Geometry check sheet. Reference: the model listing, model coordinates, mm. A direction names the side the tool comes from. Give positions to 0.01 mm unless a question says otherwise; leave off trailing zeros. Loops run counter-clockwise (first coordinate to the right, second up) from the corner with the lowest first, then second, coordinate; pieces in that order, holes last.
1. Cross-section at B-B, the plane z = 31.75. Record the cut outline in (x, y) (3 decimals).
2. Go/stop test with flat-tipped pins: pin 1 Ø1.3 at (x, z) = (-1.5, 22) entering from +Y; pin 2 Ø8 at (y, z) = (-13, 26) entering from -X; pin 3 Ø0.6 at (x, y) = (4.5, 9.5) entering from -Z; pin 4 Ø0.9 at (x, y) = (-5.5, 6) entering from +Z. Record where each tip stops, or that it passes through.
3. Tool access check on faces 1 (the flat face through (0, -17.78, -22)), 2 (the flat face through (5.25, 9, -4)), 3 (the flat face through (0, -4, 6.02)). Record the directions out of +Z, -Z, +X, -X, +Y, -Y that give a thin tool (end or side, any length) a straight path to the whole face; none if there is none.
4. Cross-section at C-C, the plane z = -31. Record the cut outline in (x, y) (3 decimals).
5. Cross-section at A-A, the plane y = 12.5. Record the cut outline in (x, z), plus the area to 3 significant figures.
6. Material ranges on L1, parallel to Z at x = -5, y = 6.5; L2, parallel to X at y = -18.6, z = 31.75, recorded low to high.
7. Cross-section at D-D, the plane y = -14.5. Record the cut outline in (x, z), plus the area to 3 significant figures.
from build123d import *

# Parameters (mm, degrees)
BOSS_EXTRUDE1_DEPTH   = 17.78
BOSS_EXTRUDE1_2_DEPTH = 17.78
BOSS_EXTRUDE1_3_DEPTH = 17.78
BOSS_EXTRUDE1_4_DEPTH = 17.78
SKETCH2_W             = 13.04
SKETCH2_H             = 12.04
BOSS_EXTRUDE2_DEPTH   = 17.78
SKETCH3_W             = 12.7
SKETCH3_H             = 76.2
SKETCH3_R             = 3.429
BOSS_EXTRUDE3_DEPTH   = 3.175
SKETCH4_OUTSIDE_W     = 32.334
SKETCH4_OUTSIDE_H     = 95.494
SKETCH4_OUTSIDE_W_2   = 12.7
SKETCH4_OUTSIDE_H_2   = 76.2
CUT_EXTRUDE2_DEPTH    = 55.722213268
CUT_EXTRUDE3_DEPTH    = 0.635


with BuildPart() as part:
    # Sketch1 → Boss-Extrude1 (new body)
    with BuildSketch(Plane(origin=(0, 0, 0), x_dir=(1, 0, 0), z_dir=(0, 1, 0))):
        Polygon((-5.25, 4.75), (-5.25, 2.718), (-6.52, 2.718), (-6.52, 6.02), (-3.218, 6.02), (-3.218, 4.75), align=None)
    extrude(amount=BOSS_EXTRUDE1_DEPTH)



with BuildPart() as body_2:
    # Sketch1 → Boss-Extrude1 2 (new body)
    with BuildSketch(Plane(origin=(0, 0, 0), x_dir=(1, 0, 0), z_dir=(0, 1, 0))):
        Polygon((6.52, 2.718), (6.52, 6.02), (3.218, 6.02), (3.218, 4.75), (5.25, 4.75), (5.25, 2.718), align=None)
    extrude(amount=BOSS_EXTRUDE1_2_DEPTH)


with BuildPart() as body_3:
    # Sketch1 → Boss-Extrude1 3 (new body)
    with BuildSketch(Plane(origin=(0, 0, 0), x_dir=(1, 0, 0), z_dir=(0, 1, 0))):
        Polygon((5.25, -2.718), (6.52, -2.718), (6.52, -6.02), (3.218, -6.02), (3.218, -4.75), (5.25, -4.75), align=None)
    extrude(amount=BOSS_EXTRUDE1_3_DEPTH)


with BuildPart() as body_4:
    # Sketch1 → Boss-Extrude1 4 (new body)
    with BuildSketch(Plane(origin=(0, 0, 0), x_dir=(1, 0, 0), z_dir=(0, 1, 0))):
        Polygon((-5.25, -2.718), (-6.52, -2.718), (-6.52, -6.02), (-3.218, -6.02), (-3.218, -4.75), (-5.25, -4.75), align=None)
    extrude(amount=BOSS_EXTRUDE1_4_DEPTH)


with BuildPart() as part_1:
    add(part.part)

    add(body_2.part)  # Boss-Extrude2 merges body 2

    add(body_3.part)  # Boss-Extrude2 merges body 3

    add(body_4.part)  # Boss-Extrude2 merges body 4
    # Sketch2 → Boss-Extrude2 (add)
    with BuildSketch(Plane(origin=(0, 0, 0), x_dir=(-1, 0, 0), z_dir=(0, -1, 0))):
        Rectangle(SKETCH2_W, SKETCH2_H)
    extrude(amount=BOSS_EXTRUDE2_DEPTH)

    # Sketch3 → Boss-Extrude3 (add)
    with BuildSketch(Plane(origin=(0, -17.78, 0), x_dir=(-1, 0, 0), z_dir=(0, -1, 0))):
        Rectangle(SKETCH3_W, SKETCH3_H)
        with Locations(Location((0, 31.75, 0), (0, 0, 90))):
            Circle(SKETCH3_R, mode=Mode.SUBTRACT)
        with Locations(Location((0, -31.75, 0), (0, 0, 270))):
            Circle(SKETCH3_R, mode=Mode.SUBTRACT)
    extrude(amount=BOSS_EXTRUDE3_DEPTH)

    # Sketch4 outside → Cut-Extrude2 (cut, through all)
    with BuildSketch(Plane.XZ.offset(20.955)):
        Rectangle(SKETCH4_OUTSIDE_W, SKETCH4_OUTSIDE_H)
        Rectangle(SKETCH4_OUTSIDE_W_2, SKETCH4_OUTSIDE_H_2, mode=Mode.SUBTRACT)
    extrude(amount=-CUT_EXTRUDE2_DEPTH, mode=Mode.SUBTRACT)

    # Sketch5 → Cut-Extrude3 (cut)
    with BuildSketch(Plane(origin=(0, -17.78, 0), x_dir=(1, 0, 0), z_dir=(0, 1, 0))):
        Polygon((-4.402938034, -19.56265828), (-3.33951656, -19.56265828), (-2.238782051, -22.073125862), (-1.138047543, -19.56265828), (-0.074626068, -19.56265828), (-1.937945713, -23.816344178), (-2.539618389, -23.816344178), align=None)
        with BuildLine():
            Line((1.380582265, -19.935788622), (0.335817308, -19.935788622))
            add(Edge.make_bspline(
                [(0.335817308, -19.935788622), (0.340329487, -19.85675768), (0.349146015, -19.702335965), (0.384215936, -19.478033479), (0.431208425, -19.266092295), (0.493926141, -19.067253807), (0.572735055, -18.881590265), (0.665607209, -18.708468733), (0.774915278, -18.5488007), (0.898332826, -18.403356174), (1.033764562, -18.272876548), (1.17839879, -18.157185114), (1.334447887, -18.061719455), (1.499060707, -17.983160056), (1.672209219, -17.920394746), (1.855531682, -17.878431057), (2.04744079, -17.850012836), (2.178818114, -17.847526128), (2.245778245, -17.846258707)],
                knots=[0, 0, 0, 0, 1.199038563, 2.342849363, 3.436047546, 4.486744587, 5.497670872, 6.488682221, 7.459191391, 8.424610317, 9.374430501, 10.305433194, 11.225809216, 12.140057399, 13.06607119, 14.010487599, 14.985989317, 16, 16, 16, 16], degree=3))
            add(Edge.make_bspline(
                [(2.245778245, -17.846258707), (2.327970856, -17.848823334), (2.488430093, -17.853830085), (2.721590093, -17.896539334), (2.93933604, -17.967977154), (3.141509653, -18.067794628), (3.326389793, -18.194602266), (3.493945801, -18.34579962), (3.639110517, -18.52455889), (3.762804328, -18.723442196), (3.865579101, -18.934031626), (3.937599381, -19.151789829), (3.984937536, -19.370938387), (3.989986444, -19.518501933), (3.992494658, -19.591809088)],
                knots=[0, 0, 0, 0, 1.075374347, 2.099382735, 3.09057751, 4.06680945, 5.040638231, 6.016817125, 7.011024321, 8.044445721, 9.0776792, 10.070479129, 11.0414456, 12, 12, 12, 12], degree=3))
            add(Edge.make_bspline(
                [(3.992494658, -19.591809088), (3.991518092, -19.636150437), (3.989552505, -19.725398619), (3.97588552, -19.860453023), (3.955382341, -19.998021723), (3.924468545, -20.137986768), (3.885916506, -20.280387391), (3.839147311, -20.425649748), (3.783076101, -20.572950255), (3.718638592, -20.723946755), (3.641764481, -20.879129473), (3.552255264, -21.04082466), (3.447735164, -21.208888878), (3.329466651, -21.384271073), (3.196875325, -21.566694641), (3.049313917, -21.755610064), (2.888481989, -21.95168302), (2.774335046, -22.082746787), (2.715689269, -22.150083995)],
                knots=[0, 0, 0, 0, 0.728284026, 1.46585585, 2.227944881, 3.01186502, 3.81876927, 4.650621989, 5.517437689, 6.406905708, 7.346299482, 8.360816762, 9.441613733, 10.596154504, 11.834900912, 13.145207542, 14.533280747, 16, 16, 16, 16], degree=3))
            Line((2.715689269, -22.150083995), (2.108186432, -22.846205289))
            Line((2.108186432, -22.846205289), (4.067120726, -22.846205289))
            Line((4.067120726, -22.846205289), (4.067120726, -23.816344178))
            Line((4.067120726, -23.816344178), (0.186565171, -23.816344178))
            Line((0.186565171, -23.816344178), (0.186565171, -23.286965505))
            Line((0.186565171, -23.286965505), (1.909960938, -21.452796668))
            add(Edge.make_bspline(
                [(1.909960938, -21.452796668), (1.959857674, -21.399293394), (2.056492855, -21.295673418), (2.193994758, -21.143496459), (2.318421835, -20.999084157), (2.427193988, -20.860898814), (2.526019439, -20.733422598), (2.610491571, -20.612813217), (2.681383236, -20.500161025), (2.758346193, -20.364322155), (2.831435702, -20.202310131), (2.898499751, -20.015665636), (2.93937993, -19.837276484), (2.945022687, -19.721034278), (2.947729701, -19.665269124)],
                knots=[0, 0, 0, 0, 1.246127091, 2.413378631, 3.493388633, 4.492180848, 5.408488754, 6.240484944, 6.999099869, 7.674939598, 8.898438119, 10.020720584, 11.050475521, 12, 12, 12, 12], degree=3))
            add(Edge.make_bspline(
                [(2.947729701, -19.665269124), (2.945705732, -19.611320641), (2.941783968, -19.506786804), (2.898686962, -19.358087978), (2.831919585, -19.223456371), (2.737834921, -19.106914927), (2.623868926, -19.011145094), (2.492170513, -18.939914183), (2.343813413, -18.898814274), (2.239812259, -18.893670033), (2.186310597, -18.891023665)],
                knots=[0, 0, 0, 0, 1.062038974, 2.057870785, 3.028805853, 4.01125022, 4.991535629, 5.949134679, 6.94496649, 8, 8, 8, 8], degree=3))
            add(Edge.make_bspline(
                [(2.186310597, -18.891023665), (2.158670957, -18.892001265), (2.104257887, -18.893925828), (2.024274927, -18.906737125), (1.948165395, -18.929315698), (1.875082148, -18.959567808), (1.80580515, -18.999667197), (1.740509141, -19.049096083), (1.678506143, -19.106598364), (1.620080529, -19.17199424), (1.566905592, -19.244976057), (1.519675807, -19.324877276), (1.480624638, -19.411648298), (1.44624257, -19.504143614), (1.419725473, -19.603356699), (1.400417737, -19.708693775), (1.385739355, -19.819983471), (1.382332567, -19.896484672), (1.380582265, -19.935788622)],
                knots=[0, 0, 0, 0, 0.903469896, 1.778625579, 2.63899355, 3.493148037, 4.358286772, 5.247621495, 6.164656832, 7.118446693, 8.109501108, 9.111810964, 10.146451449, 11.215617525, 12.33435995, 13.498009769, 14.714554818, 16, 16, 16, 16], degree=3))
        make_face()
    extrude(amount=-CUT_EXTRUDE3_DEPTH, mode=Mode.SUBTRACT)


solid = part_1.part
Result:
1. outline: (-6.35, -20.955) - (-3.429, -20.955) - (-3.429, -17.78) - (-6.35, -17.78) - close; (3.429, -20.955) - (6.35, -20.955) - (6.35, -17.78) - (3.429, -17.78) - close
2. pin 1: stops at y = -17.78
2. pin 2: passes through
2. pin 3: stops at z = -6.02
2. pin 4: stops at z = 6.02
3. face 1: -Z, +X, -X, +Y
3. face 2: +Y
3. face 3: +Z, +X, -X, +Y
4. outline: (-6.35, -20.955) - (-3.346, -20.955) - (-3.346, -17.78) - (-6.35, -17.78) - close; (3.346, -20.955) - (6.35, -20.955) - (6.35, -17.78) - (3.346, -17.78) - close
5. outline: (-6.35, -6.02) - (-3.22, -6.02) - (-3.22, -4.75) - (-5.25, -4.75) - (-5.25, -2.72) - (-6.35, -2.72) - close; (-6.35, 2.72) - (-5.25, 2.72) - (-5.25, 4.75) - (-3.22, 4.75) - (-3.22, 6.02) - (-6.35, 6.02) - close; (3.22, -6.02) - (6.35, -6.02) - (6.35, -2.72) - (5.25, -2.72) - (5.25, -4.75) - (3.22, -4.75) - close; (3.22, 4.75) - (5.25, 4.75) - (5.25, 2.72) - (6.35, 2.72) - (6.35, 6.02) - (3.22, 6.02) - close
5. area: 24.9 mm2
6. L1: z = -6.02 to -4.75, 4.75 to 6.02
6. L2: x = -6.35 to -3.43, 3.43 to 6.35
7. outline: (-6.35, -6.02) - (6.35, -6.02) - (6.35, 6.02) - (-6.35, 6.02) - close
7. area: 153 mm2
